Verification items for the finished model (mm, model axes). Face numbers are marked on the shaded views. A direction names the side the tool comes from. Coordinates: 2 decimals unless noted, no trailing zeros. Loops run counter-clockwise (first coordinate to the right, second up) from the corner with the lowest first, then second, coordinate; pieces in that order, holes last.
Q1. Sectioned sample at A-A (y = 26.5). Enter the section's corners in (x, z), then the cut area to 3 significant figures.
Q2. Sectioned sample at B-B (x = 25). Enter the section's corners in (y, z), then the cut area to 3 significant figures.
Q3. Access from +Z, -Z, +X, -X, +Y, -Y to the whole of each face (thin tool, end or side, straight path). Record for the marked faces 4 and 5.
Q4. Go/stop test with a flat-tipped pin: P1, Ø4, axis at x = 11, y = 31.5, coming from the -Z side. Record where the tip stops, or that it passes through.
Q5. Material ranges on probe 1 along X at (y, z) = (26, 5); probe 2 along Y at (x, z) = (18, 5.5); probe 3 along X at (y, z) = (11, 1.5), recorded low to high.
Q6. Sectioned sample at C-C (y = 32). Enter the section's corners in (x, z).
Q7. Mould release check, pull along X, two halves, no side actions. Record for the marked faces 1, 2 and 3: +X half, -X half, draft (parallel to the pull), parting line (faces both ways), or undercut.
Q8. Sectioned sample at D-D (z = 3.75). Enter the section's corners in (x, y) (3 decimals), then the cut area to 3 significant figures.
```python
from build123d import *

# Parameters (mm, degrees)
SKETCH1_W           = 44.45
SKETCH1_H           = 44.45
BOSS_EXTRUDE1_DEPTH = 6.35
SKETCH2_R           = 1.5
CUT_EXTRUDE2_DEPTH  = 6.35
SKETCH3_R           = 7.62
CUT_EXTRUDE3_DEPTH  = 6.35
SKETCH4_R           = 1.5
CUT_EXTRUDE4_DEPTH  = 6.35
CUT_EXTRUDE5_DEPTH  = 6.35


with BuildPart() as part:
    # Sketch1 → Boss-Extrude1 (new body)
    with BuildSketch(Plane.XY):
        with Locations((22.225, 22.225)):
            Rectangle(SKETCH1_W, SKETCH1_H)
    extrude(amount=BOSS_EXTRUDE1_DEPTH)

    # Sketch2 → Cut-Extrude2 (cut)
    with BuildSketch(Plane.XY.offset(6.35)):
        with Locations((22.225, 34.671)):
            Circle(SKETCH2_R)
        with Locations((22.225, 9.671)):
            Circle(SKETCH2_R)
    extrude(amount=-CUT_EXTRUDE2_DEPTH, mode=Mode.SUBTRACT)

    # Sketch3 → Cut-Extrude3 (cut)
    with BuildSketch(Plane.XY.offset(6.35)):
        with Locations((22.225, 22.225)):
            Circle(SKETCH3_R)
    extrude(amount=-CUT_EXTRUDE3_DEPTH, mode=Mode.SUBTRACT)

    # Sketch4 → Cut-Extrude4 (cut)
    with BuildSketch(Plane.XY.offset(6.35)):
        with Locations((3.175, 41.275)):
            Circle(SKETCH4_R)
        with Locations((41.275, 41.275)):
            Circle(SKETCH4_R)
        with Locations((41.275, 3.175)):
            Circle(SKETCH4_R)
        with Locations((3.175, 3.175)):
            Circle(SKETCH4_R)
    extrude(amount=-CUT_EXTRUDE4_DEPTH, mode=Mode.SUBTRACT)

    # Sketch7 → Cut-Extrude5 (cut)
    with BuildSketch(Plane.XY.offset(6.35)):
        with BuildLine():
            Line((38.1, 34.925), (38.1, 9.525))
            Line((38.1, 9.525), (26.437113484, 15.875))
            ThreePointArc((26.437113484, 15.875), (29.845, 22.225), (26.437113484, 28.575))
            Line((26.437113484, 28.575), (38.1, 34.925))
        make_face()
        with BuildLine():
            Line((6.35, 9.525), (18.012886516, 15.875))
            ThreePointArc((18.012886516, 15.875), (14.605, 22.225), (18.012886516, 28.575))
            Line((18.012886516, 28.575), (6.35, 34.925))
            Line((6.35, 34.925), (6.35, 9.525))
        make_face()
    extrude(amount=-CUT_EXTRUDE5_DEPTH, mode=Mode.SUBTRACT)


solid = part.part
```
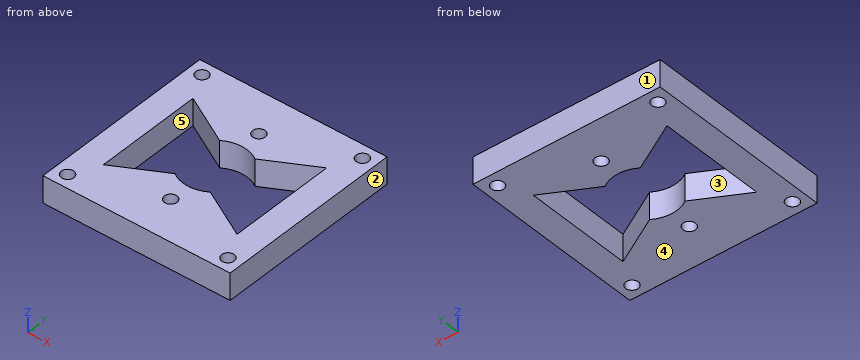
Geometry check:
1. outline: (0, 0) - (6.35, 0) - (6.35, 6.35) - (0, 6.35) - close; (38.1, 0) - (44.45, 0) - (44.45, 6.35) - (38.1, 6.35) - close
1. area: 80.6 mm2
2. outline: (0, 0) - (15.13, 0) - (15.13, 6.35) - (0, 6.35) - close; (29.32, 0) - (44.45, 0) - (44.45, 6.35) - (29.32, 6.35) - close
2. area: 192 mm2
3. face 4: -Z, +X, -X, +Y, -Y
3. face 5: +Z, -Z
4. P1: stops at z = 0
5. probe 1: x = 0 to 6.35, 38.1 to 44.45
5. probe 2: y = 0 to 15.87, 28.58 to 44.45
5. probe 3: x = 0 to 6.35, 9.06 to 21.53, 22.92 to 35.39, 38.1 to 44.45
6. outline: (0, 0) - (6.35, 0) - (6.35, 6.35) - (0, 6.35) - close; (11.72, 0) - (32.73, 0) - (32.73, 6.35) - (11.72, 6.35) - close; (38.1, 0) - (44.45, 0) - (44.45, 6.35) - (38.1, 6.35) - close
7. face 1: draft
7. face 2: +X half
7. face 3: undercut
8. outline: (0, 0) - (44.45, 0) - (44.45, 44.45) - (0, 44.45) - close; hole circle Ø3 at (3.175, 3.175); hole circle Ø3 at (3.175, 41.275); hole (6.35, 9.525) - (18.013, 15.875) arc R7.62 ccw to (26.437, 15.875) - (38.1, 9.525) - (38.1, 34.925) - (26.437, 28.575) arc R7.62 ccw to (18.013, 28.575) - (6.35, 34.925) - close; hole circle Ø3 at (22.225, 9.671); hole circle Ø3 at (22.225, 34.671); hole circle Ø3 at (41.275, 3.175); hole circle Ø3 at (41.275, 41.275)
8. area: 1,370 mm2
